from build123d import *

# Parameters (mm, degrees)
IZIM1_W                     = 50
IZIM1_H                     = 56
Y_KSEKLIK_EKSTR_ZYON1_DEPTH = 16
IZIM1_3_W                   = 39
IZIM1_3_H                   = 56
Y_KSEKLIK_EKSTR_ZYON2_DEPTH = 12
RADYUS1_R                   = 10
IZIM2_R                     = 5
KES_EKSTR_ZYON1_DEPTH       = 13
IZIM3_R                     = 5
KES_EKSTR_ZYON2_DEPTH       = 13
IZIM4_W                     = 38
IZIM4_H                     = 4
KES_EKSTR_ZYON4_DEPTH       = 57


with BuildPart() as part:
    # Çizim1 → Yükseklik-Ekstrüzyon1 (new body)
    with BuildSketch(Plane(origin=(0, 0, 0), x_dir=(1, 0, 0), z_dir=(0, 1, 0))):
        with Locations((-25, 28)):
            Rectangle(IZIM1_W, IZIM1_H)
    extrude(amount=Y_KSEKLIK_EKSTR_ZYON1_DEPTH)

    # Çizim1<3> → Yükseklik-Ekstrüzyon2 (add)
    with BuildSketch(Plane(origin=(0, 0, 0), x_dir=(1, 0, 0), z_dir=(0, 1, 0))):
        with Locations((-69.5, 28)):
            Rectangle(IZIM1_3_W, IZIM1_3_H)
        with Locations((19.5, 28)):
            Rectangle(IZIM1_3_W, IZIM1_3_H)
    extrude(amount=Y_KSEKLIK_EKSTR_ZYON2_DEPTH)

    # Radyus1
    radyus1_edges = [part.edges().sort_by_distance(p)[0] for p in [
        (-89, 6, -56),
        (-89, 6, 0),
        (39, 6, 0),
        (39, 6, -56),
    ]]
    fillet(radyus1_edges, radius=RADYUS1_R)

    # Çizim2 → Kes-Ekstrüzyon1 (cut, through all)
    with BuildSketch(Plane(origin=(0, 12, 0), x_dir=(1, 0, 0), z_dir=(0, 1, 0))):
        with Locations((-79, 46)):
            Circle(IZIM2_R)
        with Locations((-79, 10)):
            Circle(IZIM2_R)
    extrude(amount=-KES_EKSTR_ZYON1_DEPTH, mode=Mode.SUBTRACT)

    # Çizim3 → Kes-Ekstrüzyon2 (cut, through all)
    with BuildSketch(Plane(origin=(0, 12, 0), x_dir=(1, 0, 0), z_dir=(0, 1, 0))):
        with Locations((29, 46)):
            Circle(IZIM3_R)
        with Locations((29, 10)):
            Circle(IZIM3_R)
    extrude(amount=-KES_EKSTR_ZYON2_DEPTH, mode=Mode.SUBTRACT)

    # Çizim4 → Kes-Ekstrüzyon4 (cut, through all)
    with BuildSketch(Plane.XY):
        with Locations((-25, 2)):
            Rectangle(IZIM4_W, IZIM4_H)
    extrude(amount=-KES_EKSTR_ZYON4_DEPTH, mode=Mode.SUBTRACT)


solid = part.part
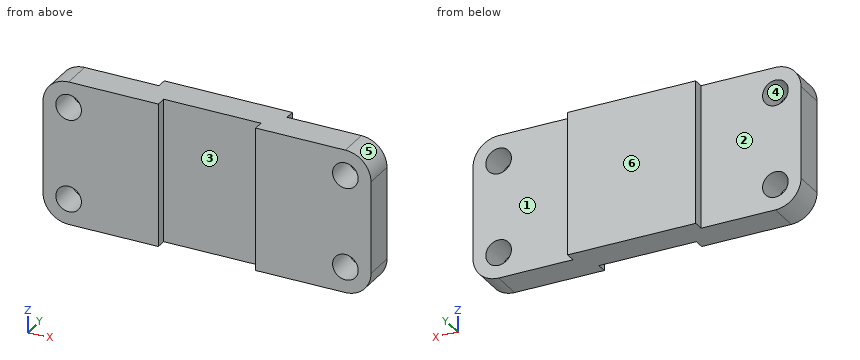
Can you work these out from the model? Positions are in its coordinate system, mm. Face numbers are marked on the shaded views. A direction names the side the tool comes from. Coordinates: 2 decimals unless noted, no trailing zeros. Loops run counter-clockwise (first coordinate to the right, second up) from the corner with the lowest first, then second, coordinate; pieces in that order, holes last. Notation, with made-up numbers: (37.25, 39) - (43.25, 39) arc R8 cw to (43.25, 54) - close; hole circle Ø3 at (43, -27). An arc over 180 degrees is marked (long way). Answer as a JSON object with one key per item and string values. Group by question number.
Item 1: On a 3-axis mill with a long thin cutter (end or side, diameter ignored), from which of +Z, -Z, +X, -X, +Y, -Y can I reach the whole of each face in a straight line? I mean the marked faces 1, 2 and 3. Say none if no direction works.
Item 2: If we section it at B-B (y = 13.5): List the corners of the cut face in (x, z) for me.
Item 3: If we section it at A-A (z = -19): List the corners of the cut face in (x, y) for me, plus the area to 3 significant figures.
Item 4: If I drill on L1, parallel to Z at x = 29, y = 6; L2, parallel to X at y = 6.75, z = -46; L3, parallel to X at y = 3.5, z = -28, over which ranges is the centre line in solid material (lowest first)? Write a range as from..to.
Item 5: For pin 1 (8 mm diameter, centred on x = 7.5, z = -10, fed in from +Y); pin 2 (2 mm diameter, centred on y = 14.5, z = -21.5, fed in from +X); pin 3 (1.2 mm diameter, centred on y = 13.5, z = -24.5, fed in from -X), each with a flat end and sliding along its axis, tell me the tip position at first contact or that it passes through.
Item 6: If we section it at C-C (x = -20): List the corners of the cut face in (y, z) for me.
Item 7: If we mould it in two halves opening along X, with no side actions, what happens to the marked faces 4, 5 and 6? For each: released by +X, released by -X, zero draft, split by the parting line, or undercut.
Returned:
{
 "1": {"face 1": "+Z, -Z, +X, +Y", "face 2": "+Z, -Z, -X, +Y", "face 3": "+Z, -Z, -Y"},
 "2": {"outline": "(-50, -56) - (0, -56) - (0, 0) - (-50, 0) - close"},
 "3": {"outline": "(-89, 0) - (-44, 0) - (-44, 4) - (-6, 4) - (-6, 0) - (39, 0) - (39, 12) - (0, 12) - (0, 16) - (-50, 16) - (-50, 12) - (-89, 12) - close", "area": "1,580 mm²"},
 "4": {"L1": "z = -56..-51, -41..-15, -5..0", "L2": "x = -89..-84, -74..24, 34..39", "L3": "x = -89..-44, -6..39"},
 "5": {"pin 1": "stops at y = 12", "pin 2": "stops at x = 0", "pin 3": "stops at x = -50"},
 "6": {"outline": "(4, -56) - (16, -56) - (16, 0) - (4, 0) - close"},
 "7": {"face 4": "undercut", "face 5": "released by +X", "face 6": "zero draft"}
}
